Can you work these out from the model? Positions are in its coordinate system, mm. A direction names the side the tool comes from. Give positions to 0.01 mm unless a question says otherwise; leave off trailing zeros. Write each loop counter-clockwise with the first axis right and the second up, starting at its lowest first coordinate (ties: lowest second). Pieces come first, ordered by that corner, then holes.
Solid Edge part; units mm, degrees
sketch "Sketch1" plane through (0, 0, 0) normal (0, -1, 0) x (1, 0, 0)
  line L0 (7, 6.8049) -> (7, 17.6049)
  line L1 (7, 17.6049) -> (10, 17.6049)
  arc A0 (10, 17.6049) -> (-10, 17.6049) centre (0, -0.1626) cw
  line L2 (-10, 17.6049) -> (-7, 17.6049)
  line L3 (-7, 17.6049) -> (-7, 6.8049)
  line L4 (-7, 6.8049) -> (7, 6.8049)
  circle A1 centre (13, 0) radius 5
  circle A2 centre (0, 0) radius 5
  circle A3 centre (6.5, -11) radius 5
  circle A4 centre (-13, 0) radius 5
  circle A5 centre (-6.5, -11) radius 5
extrude "Protrusion1" add sketch "Sketch1" along normal blind 30
sketch "Sketch2" plane through (0, 0, -1.473) normal (0, 1, 0) x (-1, 0, 0)
  line L0 (0, 23.078) -> (-10.9985, 23.078)
  arc A0 (-10.9985, 23.078) -> (10.9985, 23.078) centre (0, 1.3104) ccw
  line L1 (10.9985, 23.078) -> (0, 23.078)
  line L2 (-35, 26.723) -> (35, 26.723)
  line L3 (35, 26.723) -> (35, -23.777)
  line L4 (35, -23.777) -> (-35, -23.777)
  line L5 (-35, -23.777) -> (-35, 26.723)
extrude "Protrusion2" add sketch "Sketch2" against normal blind 30
sketch "Sketch3" plane through (0, 0, 0) normal (0, -1, 0) x (1, 0, 0)
  line L0 (35, 25.25) -> (-35, 25.25)
  line L1 (-35, 25.25) -> (-35, -25.25)
  line L2 (-35, -25.25) -> (35, -25.25)
  line L3 (35, -25.25) -> (35, 25.25)
extrude "Protrusion3" add sketch "Sketch3" against normal blind 30
sketch "Sketch4" plane through (0, 30, 0) normal (0, 1, 0) x (-1, 0, 0)
  circle A0 centre (0, 12.2049) radius 9.5
extrude "Cutout1" cut sketch "Sketch4" against normal blind 30
sketch "Sketch5" plane through (0, 30, 0) normal (0, 1, 0) x (-1, 0, 0)
  line L0 (35, -28.25) -> (-35, -28.25)
  line L1 (-35, -28.25) -> (-35, -25.25)
  line L2 (-35, -25.25) -> (35, -25.25)
  line L3 (35, -25.25) -> (35, -28.25)
extrude "Protrusion4" add sketch "Sketch5" against normal blind 76.5
sketch "Sketch6" plane through (35, -8.25, -1.5) normal (1, 0, 0) x (0, 1, 0)
  line L0 (-21.75, 26.75) -> (-21.75, -23.75)
  line L1 (-21.75, -23.75) -> (-38.25, -23.75)
  line L2 (-38.25, -23.75) -> (-38.25, -26.75)
  line L3 (-38.25, -26.75) -> (38.25, -26.75)
  line L4 (38.25, -26.75) -> (38.25, 26.75)
  line L5 (38.25, 26.75) -> (-21.75, 26.75)
extrude "Protrusion5" add sketch "Sketch6" along normal blind 10
sketch "Sketch7" plane through (-35, -8.25, -1.5) normal (-1, 0, 0) x (0, -1, 0)
  line L0 (21.75, -23.75) -> (21.75, 26.75)
  line L1 (21.75, 26.75) -> (-38.25, 26.75)
  line L2 (-38.25, 26.75) -> (-38.25, -26.75)
  line L3 (-38.25, -26.75) -> (38.25, -26.75)
  line L4 (38.25, -26.75) -> (38.25, -23.75)
  line L5 (38.25, -23.75) -> (21.75, -23.75)
extrude "Protrusion6" add sketch "Sketch7" along normal blind 10
1) If we mould it in two halves opening along X, with no side actions, what happens to faces 6 (the face through (1, 0, 25.25)), 7 (the face through (-45, 0, -1)), 8 (the face through (-4.384, 15.21, 3.777)), 9 (the face through (-1.08, -14.79, 4.88))? For each: +X half, -X half, draft (parallel to the pull), parting line (faces both ways), or undercut.
Values follow:
face 6: draft
face 7: -X half
face 8: undercut
face 9: undercut
2) For pin 1 Ø16 at (x, z) = (13, 0) entering from -Y; pin 2 Ø5 at (x, z) = (-5.5, -9) entering from -Y, each with a flat end and sliding along its axis, tell me the tip position at first contact or that it passes through.
Values follow:
pin 1: stops at y = -30
pin 2: stops at y = 0
3) For faces 1 (the face through (1, -46.5, -27)), 2 (the face through (0, 0, 6)), 3 (the face through (13, 0, 0)), 4 (the face through (1, -38, -25.25)), 5 (the face through (0, -15, 6.805)), which set-ups out of +Z, -Z, +X, -X, +Y, -Y let a thin tool reach every point of the face, with its end or its side?
Values follow:
face 1: +Z, -Z, +X, -X, -Y
face 2: +Y
face 3: -Y
face 4: +Z, +X, -X, -Y
face 5: +Y, -Y
4) Suppose I cut it at B-B on x = 0. Write out the boundary of the cut face in (y, z) (3 decimals), plus the area to 3 significant figures.
Values follow:
outline: (-46.5, -28.25) - (30, -28.25) - (30, 2.705) - (0, 2.705) - (0, -5) - (-30, -5) - (-30, -20.551) - (0, -20.551) - (0, -24.551) - (-30, -24.551) - (-30, -25.25) - (-46.5, -25.25) - close; (-30, 5) - (0, 5) - (0, 6.805) - (-30, 6.805) - close; (-30, 21.605) - (0, 21.605) - (0, 21.705) - (30, 21.705) - (30, 25.25) - (-30, 25.25) - close
area: 1,830 mm2
5) Suppose I cut it at D-D on z = 0. Write out the boundary of the cut face in (x, y).
Values follow:
outline: (-45, -30) - (-24.39, -30) - (-24.39, 0) - (-20.39, 0) - (-20.39, -30) - (-18, -30) - (-18, 0) - (-8, 0) - (-8, -30) - (-5, -30) - (-5, 0) - (5, 0) - (5, -30) - (8, -30) - (8, 0) - (18, 0) - (18, -30) - (20.39, -30) - (20.39, 0) - (24.39, 0) - (24.39, -30) - (45, -30) - (45, 30) - (-45, 30) - close
6) Suppose I cut it at A-A on y = -19.5. State how many separate pieces and enclosed holes the cut face has, plus the area to 3 significant figures.
Values follow:
separate pieces: 2
enclosed holes: 6
area: 3,710 mm2
7) Please list where these lines run through material, in increasing order: L1, parallel to Z at x = -13, y = -15; L2, parallel to Z at x = -6.5, y = -7.75 (3 decimals); L3, parallel to X at y = -17, z = 8.5.
Values follow:
L1: z = -28.25 to -20.8, -15.87 to -5, 5 to 15.54, 20.47 to 25.25
L2: z = -28.25 to -23.669, -19.487 to -16, -6 to 6.805, 21.605 to 25.25
L3: x = -45 to -22.8, -18.46 to -7, 7 to 18.46, 22.8 to 45
8) Suppose I cut it at C-C on y = 18.5. Write out the boundary of the cut face in (x, z), plus the area to 3 significant figures.
Values follow:
outline: (-45, -28.25) - (45, -28.25) - (45, 25.25) - (-45, 25.25) - close; hole circle Ø19 at (0, 12.2)
area: 4,530 mm2
